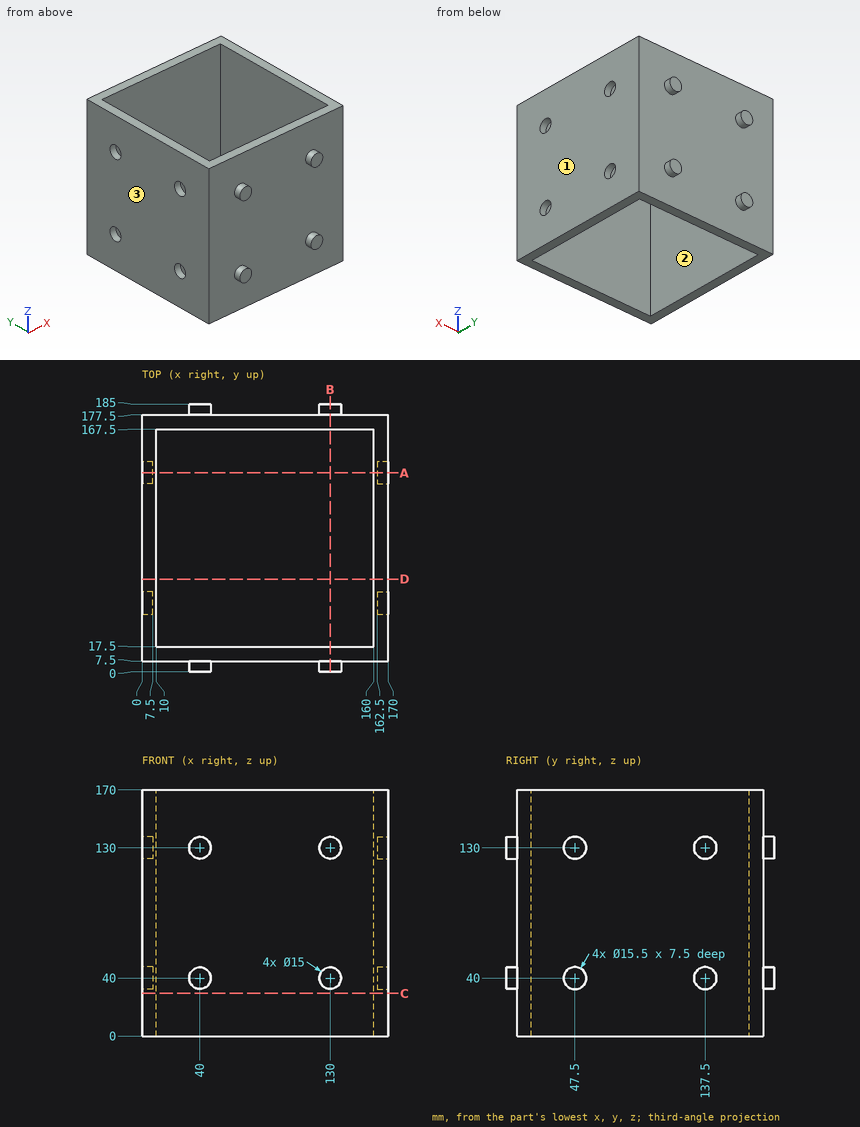
Input: dimensioned drawing with shaded views. Units: mm. Origin: part minimum x, y, z. Coordinates: 2 decimals unless noted, no trailing zeros. Order: outer loops, then holes, each group sorted by start corner. A loop starts at its lowest first (then second) coordinate and runs counter-clockwise, first axis right, second up. Notation, with made-up numbers: (-24.75, 40) - (-9.75, 40) arc R20 cw to (-9.75, 63) - close; hole circle Ø9 at (-36, 14). An arc over 180 degrees is marked (long way). Return JSON: item names as keys, results as strings. Group by question number.
1. Pin query (flat end, axial travel): pin 1 (3 mm diameter, centred on x = 99, z = 43, fed in from -Y); pin 2 (4.5 mm diameter, centred on y = 45.5, z = 40, fed in from -X); pin 3 (9.5 mm diameter, centred on y = 47.5, z = 40, fed in from +X). Return the tip coordinate at first contact, or that it passes through.
2. Cut plane A-A (y = 137.5). Output: boundary loops of the cut face in (x, z), plus the area to 4 significant figures.
3. Cut plane B-B (x = 130). Output: boundary loops of the cut face in (y, z).
4. Cut plane C-C (z = 29.5). Output: boundary loops of the cut face in (x, y), plus the area to 3 significant figures.
5. Cut plane D-D (y = 64). Output: boundary loops of the cut face in (x, z).
6. Pull-direction query (X, two-part tool) for the marked faces 1, 2 and 3; classes: pulls with the +X half, pulls with the -X half, needs draft (parallel to the pull), parting line crosses it, or undercut.
7. Material intervals for line 1 along Z through (x, y) = (4.5, 47.5); line 2 along Y through (x, z) = (116.5, 28); line 3 along X through (y, z) = (106.5, 141.5), sorted ascending. Write a range as [from, to].
Resolved:
{
 "1": {"pin 1": "stops at y = 7.5", "pin 2": "stops at x = 7.5", "pin 3": "stops at x = 162.5"},
 "2": {"outline": "(0, 0) - (10, 0) - (10, 170) - (0, 170) - (0, 137.75) - (7.5, 137.75) - (7.5, 122.25) - (0, 122.25) - (0, 47.75) - (7.5, 47.75) - (7.5, 32.25) - (0, 32.25) - close; (160, 0) - (170, 0) - (170, 32.25) - (162.5, 32.25) - (162.5, 47.75) - (170, 47.75) - (170, 122.25) - (162.5, 122.25) - (162.5, 137.75) - (170, 137.75) - (170, 170) - (160, 170) - close", "area": "2,935 mm²"},
 "3": {"outline": "(0, 32.5) - (7.5, 32.5) - (7.5, 0) - (17.5, 0) - (17.5, 170) - (7.5, 170) - (7.5, 137.5) - (0, 137.5) - (0, 122.5) - (7.5, 122.5) - (7.5, 47.5) - (0, 47.5) - close; (167.5, 0) - (177.5, 0) - (177.5, 32.5) - (185, 32.5) - (185, 47.5) - (177.5, 47.5) - (177.5, 122.5) - (185, 122.5) - (185, 137.5) - (177.5, 137.5) - (177.5, 170) - (167.5, 170) - close"},
 "4": {"outline": "(0, 7.5) - (170, 7.5) - (170, 177.5) - (0, 177.5) - close; hole (10, 17.5) - (160, 17.5) - (160, 167.5) - (10, 167.5) - close", "area": "6,400 mm²"},
 "5": {"outline": "(0, 0) - (10, 0) - (10, 170) - (0, 170) - close; (160, 0) - (170, 0) - (170, 170) - (160, 170) - close"},
 "6": {"face 1": "pulls with the +X half", "face 2": "undercut", "face 3": "pulls with the -X half"},
 "7": {"line 1": "z = [0, 32.25], [47.75, 122.25], [137.75, 170]", "line 2": "y = [7.5, 17.5], [167.5, 177.5]", "line 3": "x = [0, 10], [160, 170]"}
}
